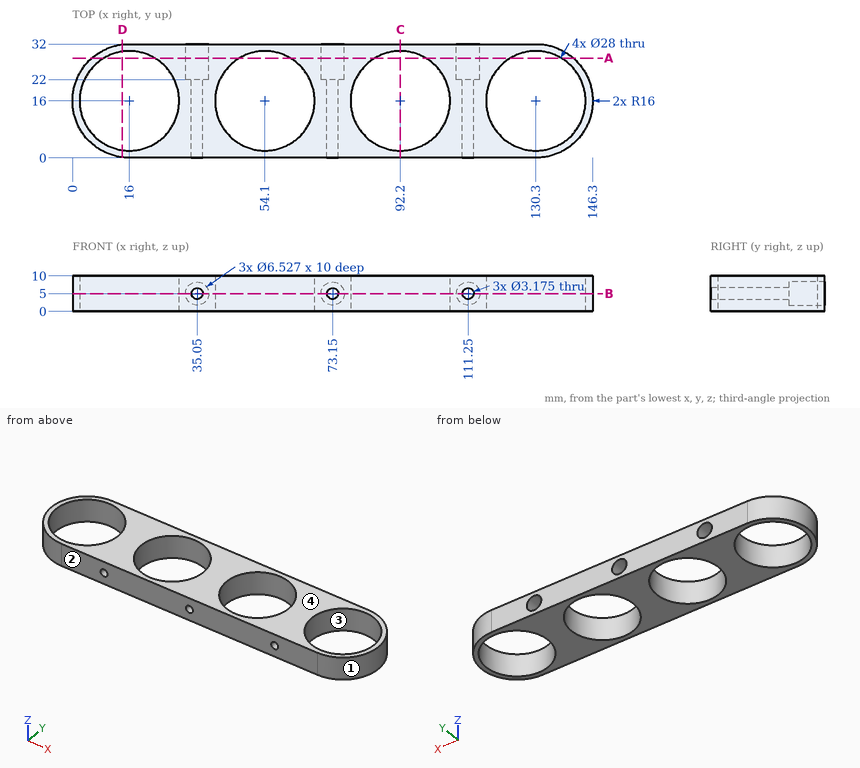
Geometry check sheet. Reference: drawing and pictorial views, mm from the part's lowest x, y, z. Give positions to 0.01 mm unless a question says otherwise; leave off trailing zeros. Write each loop counter-clockwise with the first axis right and the second up, starting at its lowest first coordinate (ties: lowest second). Pieces come first, ordered by that corner, then holes. Notation, with made-up numbers: M 53,54.5 L 61,54.5 A32 cw 61,80.5 Z; hole C 56.5,83 d11. An arc over 180 degrees is marked long. Answer as CSV lines item,"result". Start each with the question number.
Q1. Release check for a two-part mould opening along Y. For the marked faces 1, 2, 3 and 4 record: pulls with the +Y half, pulls with the -Y half, needs draft (parallel to the pull), parting line crosses it, or undercut.
Q2. Section check C-C, the plane x = 92.2. Record the cut outline in (y, z), then the cut area to 3 significant figures.
Q3. Section check D-D, the plane x = 14. Record the cut outline in (y, z).
Q4. Section check A-A, the plane y = 28. Record the cut outline in (x, z), then the cut area to 3 significant figures.
Q5. Section check B-B, the plane z = 5. Give the number of separate pieces and of enclosed holes in the cut face, then the cut area to 3 significant figures.
Q6. Material ranges on L1, parallel to Z at x = 111.5, y = 22.5; L2, parallel to Y at x = 54.1, z = 3.75; L3, parallel to X at y = 3, z = 0.75 (1 decimal), recorded low to high.
Q7. Go/stop test with flat-tipped pins: pin 1 (3.5 mm diameter, centred on x = 35.05, z = 5, fed in from +Y); pin 2 (1.5 mm diameter, centred on y = 5, z = 4, fed in from -X). Record where each tip stops, or that it passes through.
Geometry says:
1,face 1,"parting line crosses it"
1,face 2,"pulls with the -Y half"
1,face 3,"undercut"
1,face 4,"needs draft"
2,outline,"M 0,0 L 2,0 L 2,10 L 0,10 Z; M 30,0 L 32,0 L 32,10 L 30,10 Z"
2,area,"40.0 mm^2"
3,outline,"M 0.13,0 L 2.14,0 L 2.14,10 L 0.13,10 Z; M 29.86,0 L 31.87,0 L 31.87,10 L 29.86,10 Z"
4,outline,"M 5.42,0 L 8.79,0 L 8.79,10 L 5.42,10 Z; M 23.21,0 L 46.89,0 L 46.89,10 L 23.21,10 Z; M 61.31,0 L 84.99,0 L 84.99,10 L 61.31,10 Z; M 99.41,0 L 123.09,0 L 123.09,10 L 99.41,10 Z; M 137.51,0 L 140.88,0 L 140.88,10 L 137.51,10 Z; hole C 35.05,5 d6.53; hole C 73.15,5 d6.53; hole C 111.25,5 d6.53"
4,area,"677 mm^2"
5,separate pieces,"4"
5,enclosed holes,"4"
5,area,"1,590 mm^2"
6,L1,"0 to 1.75, 8.25 to 10"
6,L2,"0 to 2, 30 to 32"
6,L3,"6.7 to 10.8, 21.2 to 48.9, 59.3 to 87, 97.4 to 125.1, 135.5 to 139.6"
7,pin 1,"y = 22"
7,pin 2,"x = 3.71"
